Build history of the part. All positions in model axes, mm. Coordinates: 2 decimals unless noted, no trailing zeros. Order: outer loops, then holes, each group sorted by start corner. A loop starts at its lowest first (then second) coordinate and runs counter-clockwise, first axis right, second up. Notation, with made-up numbers: (17, 50) - (30, 50) arc R23 cw to (30, 78) - close; hole circle Ø2 at (62, -16.5). An arc over 180 degrees is marked (long way). Answer as CSV lines item,"result". Start each with the question number.
from build123d import *

# Parameters (mm, degrees)
SKETCH1_R           = 2
SKETCH1_R_2         = 2.55
BOSS_EXTRUDE2_DEPTH = 3


with BuildPart() as part:
    # Sketch1 → Boss-Extrude2 (new body)
    with BuildSketch(Plane(origin=(0, 0, 0), x_dir=(1, 0, 0), z_dir=(0, 1, 0))):
        with BuildLine():
            Line((-37, 15), (37, 15))
            ThreePointArc((37, 15), (39.121320344, 14.121320344), (40, 12))
            Line((40, 12), (40, -12))
            ThreePointArc((40, -12), (39.121320344, -14.121320344), (37, -15))
            Line((37, -15), (-37, -15))
            ThreePointArc((-37, -15), (-39.121320344, -14.121320344), (-40, -12))
            Line((-40, -12), (-40, 12))
            ThreePointArc((-40, 12), (-39.121320344, 14.121320344), (-37, 15))
        make_face()
        with Locations((20.5, 6.8)):
            Circle(SKETCH1_R, mode=Mode.SUBTRACT)
        with Locations((31.5, 6.8)):
            Circle(SKETCH1_R, mode=Mode.SUBTRACT)
        with Locations((-30, 6)):
            Circle(SKETCH1_R_2, mode=Mode.SUBTRACT)
        with Locations((-30, -6)):
            Circle(SKETCH1_R_2, mode=Mode.SUBTRACT)
        with Locations((-7.5, 6)):
            Circle(SKETCH1_R_2, mode=Mode.SUBTRACT)
        with Locations((-7.5, -6)):
            Circle(SKETCH1_R_2, mode=Mode.SUBTRACT)
    extrude(amount=BOSS_EXTRUDE2_DEPTH)


solid = part.part
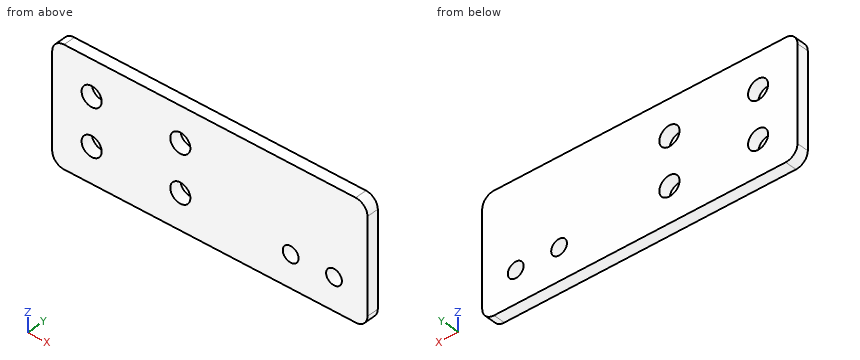
(1) Band-saw the part on A-A on y = 0.6. List the corners of the cut face in (x, z), plus the area to 3 significant figures.
(2) Band-saw the part on C-C on z = 6. List the corners of the cut face in (x, y).
(3) Band-saw the part on D-D on x = -30. List the corners of the cut face in (y, z), plus the area to 3 significant figures.
(4) Drop a flat-ended pin along its axis: pin 1 Ø4.5 at (x, z) = (-30, -6) entering from -Y. Give the stop position or say it passes through.
(5) Probe L1, parallel to X at y = 1.2, z = 6; L2, parallel to Z at x = -30, y = 0.75; L3, parallel to Z at x = 20.5, y = 0.9. List the from-to ranges inside material, lowest first. Write a range as [from, to].
(6) Band-saw the part on B-B on x = 31.5. List the corners of the cut face in (y, z), plus the area to 3 significant figures.
Filled in:
1,outline,"(-40, -12) arc R3 ccw to (-37, -15) - (37, -15) arc R3 ccw to (40, -12) - (40, 12) arc R3 ccw to (37, 15) - (-37, 15) arc R3 ccw to (-40, 12) - close; hole circle Ø5.1 at (-30, -6); hole circle Ø5.1 at (-30, 6); hole circle Ø5.1 at (-7.5, -6); hole circle Ø5.1 at (-7.5, 6); hole circle Ø4 at (20.5, -6.8); hole circle Ø4 at (31.5, -6.8)"
1,area,"2,290 mm^2"
2,outline,"(-40, 0) - (-32.55, 0) - (-32.55, 3) - (-40, 3) - close; (-27.45, 0) - (-10.05, 0) - (-10.05, 3) - (-27.45, 3) - close; (-4.95, 0) - (40, 0) - (40, 3) - (-4.95, 3) - close"
3,outline,"(0, -15) - (3, -15) - (3, -8.55) - (0, -8.55) - close; (0, -3.45) - (3, -3.45) - (3, 3.45) - (0, 3.45) - close; (0, 8.55) - (3, 8.55) - (3, 15) - (0, 15) - close"
3,area,"59.4 mm^2"
4,pin 1,"passes through"
5,L1,"x = [-40, -32.55], [-27.45, -10.05], [-4.95, 40]"
5,L2,"z = [-15, -8.55], [-3.45, 3.45], [8.55, 15]"
5,L3,"z = [-15, -8.8], [-4.8, 15]"
6,outline,"(0, -15) - (3, -15) - (3, -8.8) - (0, -8.8) - close; (0, -4.8) - (3, -4.8) - (3, 15) - (0, 15) - close"
6,area,"78.0 mm^2"
